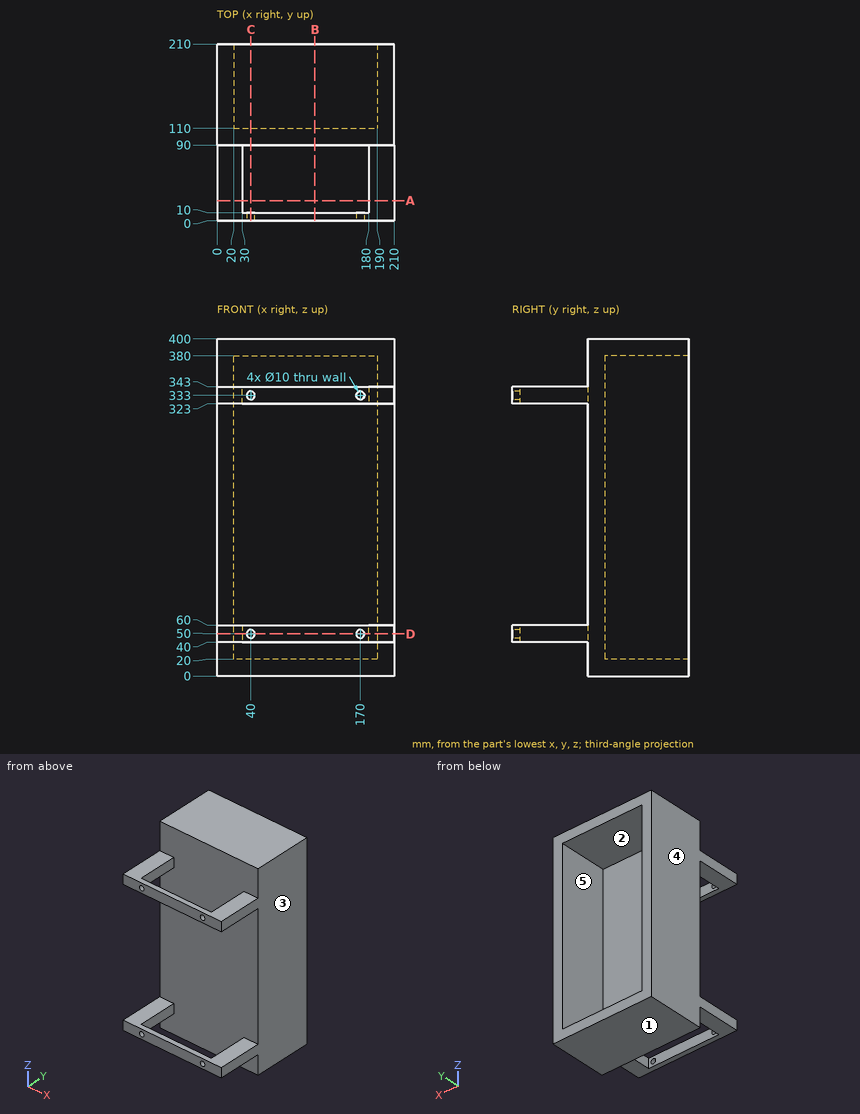
Could you check a few things on this drawing? It's one solid part, dimensions in mm from its lowest x, y, z. A direction names the side the tool comes from. Round coordinates to 2 decimals unless told otherwise and drop trailing zeros. Order: outer loops, then holes, each group sorted by start corner. A loop starts at its lowest first (then second) coordinate and runs counter-clockwise, first axis right, second up. Notation, with made-up numbers: (-34.75, -38) -> (3.25, -38) arc R11 cw to (3.25, -28) -> close; hole circle Ø3 at (84, 83.5). An arc over 180 degrees is marked (long way). One line per question, with ' | ' between items.
Q1. I'm going to push flat-ended pins straight in: pin 1 (12 mm diameter, centred on x = 69, z = 112.5, fed in from +Y); pin 2 (12 mm diameter, centred on x = 186, z = 250, fed in from -Y); pin 3 (3 mm diameter, centred on x = 31, y = 27.5, fed in from -Z). Where does each tip first touch, or does it pass through?
Computed values:
pin 1: y = 110 | pin 2: y = 90 | pin 3: z = 40
Q2. If we section it at D-D on z = 50: Write out the boundary of the cut face in (x, y), plus the area to 3 significant figures.
Computed values:
outline: (0, 0) -> (35, 0) -> (35, 10) -> (30, 10) -> (30, 90) -> (180, 90) -> (180, 10) -> (175, 10) -> (175, 0) -> (210, 0) -> (210, 210) -> (190, 210) -> (190, 110) -> (20, 110) -> (20, 210) -> (0, 210) -> close; (45, 0) -> (165, 0) -> (165, 10) -> (45, 10) -> close | area: 14,900 mm²
Q3. If we section it at B-B on x = 116: Write out the boundary of the cut face in (y, z), plus the area to 3 significant figures.
Computed values:
outline: (0, 40) -> (10, 40) -> (10, 60) -> (0, 60) -> close; (0, 323) -> (10, 323) -> (10, 343) -> (0, 343) -> close; (90, 0) -> (210, 0) -> (210, 20) -> (110, 20) -> (110, 380) -> (210, 380) -> (210, 400) -> (90, 400) -> close | area: 12,400 mm²
Q4. We'd pull the mould along X, two halves only. Please class the marked faces 3, 4 and 5: released by +X, released by -X, zero draft, split by the parting line, or undercut.
Computed values:
face 3: released by +X | face 4: released by -X | face 5: undercut
Q5. If we section it at C-C on x = 40: Write out the boundary of the cut face in (y, z), plus the area to 3 significant figures.
Computed values:
outline: (0, 40) -> (10, 40) -> (10, 45) -> (0, 45) -> close; (0, 55) -> (10, 55) -> (10, 60) -> (0, 60) -> close; (0, 323) -> (10, 323) -> (10, 328) -> (0, 328) -> close; (0, 338) -> (10, 338) -> (10, 343) -> (0, 343) -> close; (90, 0) -> (210, 0) -> (210, 20) -> (110, 20) -> (110, 380) -> (210, 380) -> (210, 400) -> (90, 400) -> close | area: 12,200 mm²
Q6. If I drill on line 1 (Z direction, x = 40, y = 5); line 2 (X direction, y = 186, z = 260); line 3 (Z direction, x = 196, y = 48), over which ranges is the centre line in solid material (lowest first)? Write a range as from..to.
Computed values:
line 1: 40..45, 55..60, 323..328, 338..343 | line 2: 0..20, 190..210 | line 3: 40..60, 323..343
Q7. If we section it at A-A on y = 24: Write out the boundary of the cut face in (x, z), plus the area to 3 significant figures.
Computed values:
outline: (0, 40) -> (30, 40) -> (30, 60) -> (0, 60) -> close; (0, 323) -> (30, 323) -> (30, 343) -> (0, 343) -> close; (180, 40) -> (210, 40) -> (210, 60) -> (180, 60) -> close; (180, 323) -> (210, 323) -> (210, 343) -> (180, 343) -> close | area: 2,400 mm²
Q8. Which directions (+Z, -Z, +X, -X, +Y, -Y) give clear straight access to the entire face, cutting with the end or side of a thin tool? Please do the marked faces 1 and 2.
Computed values:
face 1: -Z, +X, -X, +Y, -Y | face 2: +Y
